Could you check a few things on this model? Use its own coordinates, in mm. Give positions to 0.01 mm unless a question says otherwise; leave off trailing zeros. Loops run counter-clockwise (first coordinate to the right, second up) from the corner with the lowest first, then second, coordinate; pieces in that order, holes last. Notation, with made-up numbers: (78.25, -16) - (120.25, -16) arc R15 cw to (120.25, -9) - close; hole circle Ø5 at (3.25, -23). An arc over 180 degrees is marked (long way). One line per item, written item: value. Start each with the question number.
Q1. If I drill on line 1 (X direction, y = -46, z = 1.55); line 2 (Y direction, x = 91, z = 0.95); line 3 (X direction, y = -9, z = 5.45), over which ranges is the centre line in solid material (lowest first)? Write a range as from..to.
Q2. I want a section at B-B (x = -132). Please give me the cut outline in (y, z).
Q3. I want a section at A-A (y = -101). Please give me the cut outline in (x, z).
Q4. I want a section at C-C (z = 3.9). Please give me the cut outline in (x, y).
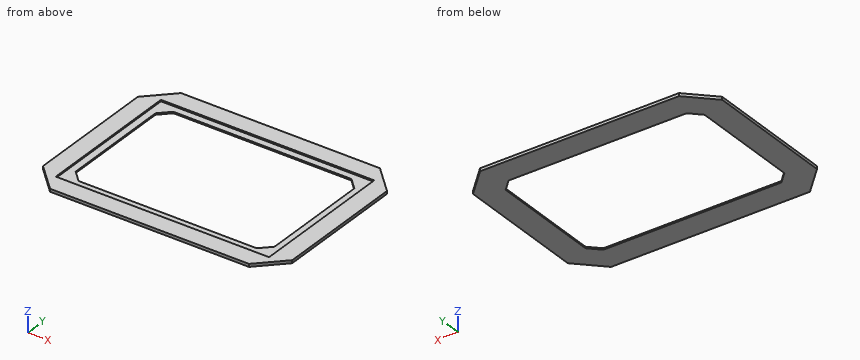
```python
from build123d import *

# Parameters (mm, degrees)
PAD_DEPTH    = 6
SKETCH001_W  = 445
SKETCH001_H  = 305
POCKET_DEPTH = 3


with BuildPart() as part:
    # Sketch → Pad (new body)
    with BuildSketch(Plane.XY):
        Polygon((-207.5, 190), (207.5, 190), (260, 137.5), (260, -137.5), (207.5, -190), (-207.5, -190), (-260, -137.5), (-260, 137.5), align=None)
        Polygon((-207.5, -115.753788), (-207.5, 115.753788), (-185.753788, 137.5), (185.753788, 137.5), (207.5, 115.753788), (207.5, -115.753788), (185.753788, -137.5), (-185.753788, -137.5), align=None, mode=Mode.SUBTRACT)
    extrude(amount=PAD_DEPTH)

    # Sketch001 (on Face18 of Pad) → Pocket (cut)
    with BuildSketch(Plane.XY.offset(6)):
        Rectangle(SKETCH001_W, SKETCH001_H)
    extrude(amount=-POCKET_DEPTH, mode=Mode.SUBTRACT)


solid = part.part
```
Worked answers:
1. line 1: x = -260..-207.5, 207.5..260
1. line 2: y = -190..-137.5, 137.5..190
1. line 3: x = -260..-222.5, 222.5..260
2. outline: (-190, 0) - (-137.5, 0) - (-137.5, 3) - (-152.5, 3) - (-152.5, 6) - (-190, 6) - close; (137.5, 0) - (190, 0) - (190, 6) - (152.5, 6) - (152.5, 3) - (137.5, 3) - close
3. outline: (-260, 0) - (-207.5, 0) - (-207.5, 3) - (-222.5, 3) - (-222.5, 6) - (-260, 6) - close; (207.5, 0) - (260, 0) - (260, 6) - (222.5, 6) - (222.5, 3) - (207.5, 3) - close
4. outline: (-260, -137.5) - (-207.5, -190) - (207.5, -190) - (260, -137.5) - (260, 137.5) - (207.5, 190) - (-207.5, 190) - (-260, 137.5) - close; hole (-222.5, -152.5) - (222.5, -152.5) - (222.5, 152.5) - (-222.5, 152.5) - close
